```python
from build123d import *

# Parameters (mm, degrees)
EXTRUDE_1_DEPTH           = 2.5
FILLET_1_R                = 3
SKETCH_2_R                = 1.775
CUT_EXTRUDE_1_DEPTH       = 1
CUT_EXTRUDE_1_DEPTH_BACK  = 6
SKETCH_4_R                = 2.025
CUT_EXTRUDE_3_DEPTH       = 1
CUT_EXTRUDE_3_DEPTH_BACK  = 6
SKETCH_12_W               = 6
SKETCH_12_H               = 3.5
CUT_EXTRUDE_9_DEPTH       = 10
SKETCH_14_W               = 20
SKETCH_14_H               = 5
EXTRUDE_3_DEPTH           = 5
CUT_EXTRUDE_10_DEPTH      = 5
CUT_EXTRUDE_START         = -6
SKETCH_16_R               = 1.525
CUT_EXTRUDE_11_DEPTH      = 7
SKETCH_18_R               = 1.525
CUT_EXTRUDE_13_DEPTH      = 8
HOLE_WIZARD_1_D           = 3
HOLE_WIZARD_1_CSINK_D     = 8
HOLE_WIZARD_1_CSINK_ANGLE = 90
SKETCH_20_R               = 1.525
CUT_EXTRUDE_14_DEPTH      = 6.0000001
SKETCH_21_R               = 14.5
CUT_EXTRUDE_15_DEPTH      = 6.0000001


with BuildPart() as part:
    # 草图1 → 凸台-拉伸1 (new body, symmetric)
    with BuildSketch(Plane(origin=(0, 0, 0), x_dir=(1, 0, 0), z_dir=(0, 1, 0))):
        with BuildLine():
            Line((0, 47.5), (80, 47.5))
            Line((80, 47.5), (80, -47.5))
            Line((80, -47.5), (0, -47.5))
            ThreePointArc((0, -47.5), (-47.5, 0), (0, 47.5))
        make_face()
    extrude(amount=EXTRUDE_1_DEPTH, both=True)

    # 圆角1
    fillet_1_edges = [part.edges().sort_by_distance(p)[0] for p in [
        (80, 0, -47.5),
        (80, 0, 47.5),
    ]]
    fillet(fillet_1_edges, radius=FILLET_1_R)

    # 草图2 → 切除-拉伸1 (cut, two sides)
    with BuildSketch(Plane(origin=(0, 2.5, 0), x_dir=(1, 0, 0), z_dir=(0, 1, 0))) as cut_extrude_1_sk:
        with Locations((-39.264880132, 16.264045876)):
            Circle(SKETCH_2_R)
        with Locations((-16.264045876, 39.264880132)):
            Circle(SKETCH_2_R)
        with Locations((16.264045876, 39.264880132)):
            Circle(SKETCH_2_R)
        with Locations((39.264880132, 16.264045876)):
            Circle(SKETCH_2_R)
        with Locations((39.264880132, -16.264045876)):
            Circle(SKETCH_2_R)
        with Locations((16.264045876, -39.264880132)):
            Circle(SKETCH_2_R)
        with Locations((-16.264045876, -39.264880132)):
            Circle(SKETCH_2_R)
        with Locations((-39.264880132, -16.264045876)):
            Circle(SKETCH_2_R)
    extrude(amount=CUT_EXTRUDE_1_DEPTH, mode=Mode.SUBTRACT)
    extrude(cut_extrude_1_sk.sketch, amount=-CUT_EXTRUDE_1_DEPTH_BACK, mode=Mode.SUBTRACT)

    # 草图4 → 切除-拉伸3 (cut, two sides)
    with BuildSketch(Plane(origin=(0, 2.5, 0), x_dir=(1, 0, 0), z_dir=(0, 1, 0))) as cut_extrude_3_sk:
        with Locations((76, -33.5)):
            Circle(SKETCH_4_R)
        with Locations((76, 33.5)):
            Circle(SKETCH_4_R)
        with Locations((76, 18.5)):
            Circle(SKETCH_4_R)
        with Locations((76, -18.5)):
            Circle(SKETCH_4_R)
    extrude(amount=CUT_EXTRUDE_3_DEPTH, mode=Mode.SUBTRACT)
    extrude(cut_extrude_3_sk.sketch, amount=-CUT_EXTRUDE_3_DEPTH_BACK, mode=Mode.SUBTRACT)

    # 草图12 → 切除-拉伸9 (cut)
    with BuildSketch(Plane(origin=(0, 2.5, 0), x_dir=(1, 0, 0), z_dir=(0, 1, 0))):
        with Locations((77, -45.75)):
            Rectangle(SKETCH_12_W, SKETCH_12_H)
    cut_extrude_9 = extrude(amount=-CUT_EXTRUDE_9_DEPTH, mode=Mode.SUBTRACT)

    # 草图14 → 凸台-拉伸3 (add)
    with BuildSketch(Plane.XY.offset(47.5)):
        with Locations((59, 0)):
            Rectangle(SKETCH_14_W, SKETCH_14_H)
        with Locations((16, 0)):
            Rectangle(SKETCH_14_W, SKETCH_14_H)
    extrude_3 = extrude(amount=EXTRUDE_3_DEPTH)

    # 草图15 → 切除-拉伸10 (cut)
    with BuildSketch(Plane(origin=(0, 2.5, 0), x_dir=(1, 0, 0), z_dir=(0, 1, 0))):
        with BuildLine():
            Line((26, -47.5), (29, -47.5))
            ThreePointArc((29, -47.5), (27.5, -46), (26, -47.5))
        make_face()
        with BuildLine():
            Line((46, -47.5), (49, -47.5))
            ThreePointArc((49, -47.5), (47.5, -46), (46, -47.5))
        make_face()
        with BuildLine():
            Line((71.5, -47.5), (69, -47.5))
            ThreePointArc((69, -47.5), (70.25, -46.829156198), (71.5, -47.5))
        make_face()
        with BuildLine():
            Line((3, -47.5), (6, -47.5))
            ThreePointArc((6, -47.5), (4.5, -46), (3, -47.5))
        make_face()
    cut_extrude_10 = extrude(amount=-CUT_EXTRUDE_10_DEPTH, mode=Mode.SUBTRACT)

    # 镜向4: 凸台-拉伸3 across plane
    add(extrude_3.mirror(Plane.XY))

    # 草图16 → 切除-拉伸11 (cut)
    with BuildSketch(Plane(origin=(0, 2.5, 0), x_dir=(1, 0, 0), z_dir=(0, 1, 0)).offset(CUT_EXTRUDE_START)):
        with Locations((34, -44.5)):
            Circle(SKETCH_16_R)
        with Locations((54, -44.5)):
            Circle(SKETCH_16_R)
    cut_extrude_11 = extrude(amount=CUT_EXTRUDE_11_DEPTH, mode=Mode.SUBTRACT)

    # 镜向5: 切除-拉伸9, 切除-拉伸10, 切除-拉伸11 across plane
    add(cut_extrude_9.mirror(Plane.XY), mode=Mode.SUBTRACT)
    add(cut_extrude_10.mirror(Plane.XY), mode=Mode.SUBTRACT)
    add(cut_extrude_11.mirror(Plane.XY), mode=Mode.SUBTRACT)

    # 草图18 → 切除-拉伸13 (cut)
    with BuildSketch(Plane(origin=(0, 2.5, 0), x_dir=(1, 0, 0), z_dir=(0, 1, 0))):
        with Locations((-3, 43.5)):
            Circle(SKETCH_18_R)
    extrude(amount=-CUT_EXTRUDE_13_DEPTH, mode=Mode.SUBTRACT)

    # 孔1 (through all)
    with Locations(Plane(origin=(-3, -2.5, -43.5), x_dir=(0, 0, -1), z_dir=(0, -1, 0))):
        with Locations((0, 0)):
            hole_wizard_1 = CounterSinkHole(HOLE_WIZARD_1_D / 2, HOLE_WIZARD_1_CSINK_D / 2, counter_sink_angle=HOLE_WIZARD_1_CSINK_ANGLE)

    # 镜向6: 孔1 across plane
    add(hole_wizard_1.mirror(Plane.XY), mode=Mode.SUBTRACT)

    # 草图20 → 切除-拉伸14 (cut, through all)
    with BuildSketch(Plane(origin=(0, 2.5, 0), x_dir=(1, 0, 0), z_dir=(0, 1, 0))):
        with Locations((-13.435028843, 13.435028843)):
            Circle(SKETCH_20_R)
        with Locations((0, 19)):
            Circle(SKETCH_20_R)
        with Locations((13.435028843, 13.435028843)):
            Circle(SKETCH_20_R)
        with Locations((19, 0)):
            Circle(SKETCH_20_R)
        with Locations((13.435028843, -13.435028843)):
            Circle(SKETCH_20_R)
        with Locations((0, -19)):
            Circle(SKETCH_20_R)
        with Locations((-13.435028843, -13.435028843)):
            Circle(SKETCH_20_R)
        with Locations((-19, 0)):
            Circle(SKETCH_20_R)
    extrude(amount=-CUT_EXTRUDE_14_DEPTH, mode=Mode.SUBTRACT)

    # 草图21 → 切除-拉伸15 (cut, through all)
    with BuildSketch(Plane.XZ.offset(2.5)):
        Circle(SKETCH_21_R)
    extrude(amount=-CUT_EXTRUDE_15_DEPTH, mode=Mode.SUBTRACT)


solid = part.part
```
Design review of the part built by this model. Coordinates are the model's own, in mm. A direction names the side the tool comes from. Give positions to 0.01 mm unless a question says otherwise; leave off trailing zeros. Order: outer loops, then holes, each group sorted by start corner. A loop starts at its lowest first (then second) coordinate and runs counter-clockwise, first axis right, second up. Notation, with made-up numbers: M -18,53.5 L -9,53.5 A14 cw -9,67.5 Z; hole C -27,40 d2. An arc over 180 degrees is marked long. One line per question, with ' | ' between items. Start each with the question number.
Q1. The part is to be moulded in two halves that separate along Z. For faces 6 (the face through (26, 0, 50)), 7 (the face through (59, 0, -52.5)), 8 (the face through (-0.33, 0.04, 20.49)), say which applies: +Z half, -Z half, draft (parallel to the pull), parting line (faces both ways), or undercut.
Q2. We need section D-D (y = -1.5). State how many separate pieces and enclosed holes the cut face has, plus the area to 3 significant figures.
Q3. Machinability: for faces 1 (the face through (73, 0, -47.5)), 2 (the face through (77.1, 0, -35.2)), 3 (the face through (37, 0, -47.5)), 4 (the face through (73, 0, 47.5)), 5 (the face through (49, 0, 50)), which of the approach directions +Z, -Z, +X, -X, +Y, -Y give a long, thin tool a straight path to every point of the face, cutting with its end or side? Answer none if there is none.
Q4. We need section B-B (z = 8.5). Write out the cut boundary in (x, y), plus the area to 3 significant figures.
Q5. We need section A-A (x = 54). Write out the cut boundary in (y, z) (3 decimals).
Q6. We need section C-C (x = 9). Write out the cut boundary in (y, z), plus the area to 3 significant figures.
Q7. For pin 1 Ø2.5 at (y, z) = (1, -50) entering from +X; pin 2 Ø1.8 at (y, z) = (-1, 46) entering from +X; pin 3 Ø1 at (x, y) = (-20, 0.5) entering from +Z, all flat-tipped, find the tip position at first contact; note any pin that passes through.
Q8. For L1, parallel to Z at x = 39, y = -1; L2, parallel to Z at x = 76, y = 1.35 (3 decimals); L3, parallel to Z at x = -3, y = 1.15 (3 decimals), list the stretches that pass through material, from the lowest coordinate up. Write a range as [from, to].
Returned:
1) face 6: draft | face 7: -Z half | face 8: undercut
2) separate pieces: 1 | enclosed holes: 27 | area: 10,500 mm2
3) face 1: -Z, +X, +Y, -Y | face 2: +Y, -Y | face 3: -Z, +Y, -Y | face 4: +Z, +X, +Y, -Y | face 5: +Z, +Y, -Y
4) outline: M -46.73,-2.5 L -11.75,-2.5 L -11.75,2.5 L -46.73,2.5 Z; M 11.75,-2.5 L 80,-2.5 L 80,2.5 L 11.75,2.5 Z | area: 516 mm2
5) outline: M -2.5,-52.5 L 2.5,-52.5 L 2.5,-46.025 L -2.5,-46.025 Z; M -2.5,-42.975 L 2.5,-42.975 L 2.5,42.975 L -2.5,42.975 Z; M -2.5,46.025 L 2.5,46.025 L 2.5,52.5 L -2.5,52.5 Z
6) outline: M -2.5,-52.5 L 2.5,-52.5 L 2.5,-11.37 L -2.5,-11.37 Z; M -2.5,11.37 L 2.5,11.37 L 2.5,52.5 L -2.5,52.5 Z | area: 411 mm2
7) pin 1: x = 69 | pin 2: x = 74 | pin 3: z = 43.31
8) L1: [-47.5, -18.02], [-14.51, 14.51], [18.02, 47.5] | L2: [-44, -35.525], [-31.475, -20.525], [-16.475, 16.475], [20.525, 31.475], [35.525, 44] | L3: [-47.405, -45.025], [-41.975, -14.186], [14.186, 42], [45, 47.405]
